```python
from build123d import *

# Parameters (mm, degrees)
F0_W     = 152.095206
F0_H     = 16.764
F1_DEPTH = 254
F2_R     = 9.455493
F2_R_2   = 9.174566
F2_R_3   = 11.28492
F2_R_4   = 9.817554
F3_DEPTH = 203.2


with BuildPart() as f1:
    # F0 (on Front) → F1 (new body)
    with BuildSketch(Plane.XZ):
        with Locations((0.609603, -1.6764)):
            Rectangle(F0_W, F0_H)
    extrude(amount=F1_DEPTH)

    # F2 (on face) → F3 (join)
    with BuildSketch(Plane(origin=(0, 0, -10.0584), x_dir=(1, 0, 0), z_dir=(0, 0, -1))):
        with Locations((-60.858399, 241.452411)):
            Circle(F2_R)
        with Locations((-60.858399, 13.614404)):
            Circle(F2_R_2)
        with Locations((57.353202, 12.954001)):
            Circle(F2_R_3)
        with Locations((56.032401, 243.43361)):
            Circle(F2_R_4)
    extrude(amount=F3_DEPTH)


solid = f1.part
```
Design review of the part built by this model. Coordinates are the model's own, in mm. A direction names the side the tool comes from. Round coordinates to 2 decimals unless told otherwise and drop trailing zeros. Write each loop counter-clockwise with the first axis right and the second up, starting at its lowest first coordinate (ties: lowest second). Pieces come first, ordered by that corner, then holes. Notation, with made-up numbers: (-2.75, 25.5) -> (53.25, 25.5) arc R15 ccw to (53.25, 39.5) -> close; hole circle Ø10 at (35, 60.5). An arc over 180 degrees is marked (long way). Answer in a Markdown table with one row per item.
Q1. Take a section at A-A, the plane x = -57.5. State the section outline as (y, z) points, then the cut area to 3 significant figures.
The answers:
| item | result |
|---|---|
| outline | (-254, -10.06) -> (-250.29, -10.06) -> (-250.29, -213.26) -> (-232.61, -213.26) -> (-232.61, -10.06) -> (-22.15, -10.06) -> (-22.15, -213.26) -> (-5.08, -213.26) -> (-5.08, -10.06) -> (0, -10.06) -> (0, 6.71) -> (-254, 6.71) -> close |
| area | 11,300 mm² |
Q2. Clearance check with flat-ended pins moving along their axes: pin 1 Ø8 at (x, y) = (27.5, -70.5) entering from -Z; pin 2 Ø12 at (y, z) = (-36, -157.5) entering from +X. State where each tip first meets the part, or that it passes through.
The answers:
| item | result |
|---|---|
| pin 1 | z = -10.06 |
| pin 2 | through |
Q3. Take a section at B-B, the plane z = -65.5. State the section outline as (x, y) points, then the cut area to 3 significant figures.
The answers:
| item | result |
|---|---|
| outline | circle Ø18.91 at (-60.86, -241.45); circle Ø18.35 at (-60.86, -13.61); circle Ø22.57 at (57.35, -12.95); circle Ø19.64 at (56.03, -243.43) |
| area | 1,250 mm² |
Q4. For faces 1 (the face through (-52, -16, -110)), 2 (the face through (0, -254, -2)), list the 3-axis set-ups (+Z, -Z, +X, -X, +Y, -Y) from which the entire face can be reached by the end or side of a thin tool; tool diameter is ignored.
The answers:
| item | result |
|---|---|
| face 1 | -Z |
| face 2 | +Z, -Z, +X, -X, -Y |
Q5. Take a section at D-D, the plane x = 23.5. State the section outline as (y, z) points.
The answers:
| item | result |
|---|---|
| outline | (-254, -10.06) -> (0, -10.06) -> (0, 6.71) -> (-254, 6.71) -> close |
Q6. Take a section at C-C, the plane y = -224. State the section outline as (x, z) points.
The answers:
| item | result |
|---|---|
| outline | (-75.44, -10.06) -> (76.66, -10.06) -> (76.66, 6.71) -> (-75.44, 6.71) -> close |
Q7. To check wall thickness, follow L1, parallel to Z at x = -39, y = -106; L2, parallel to Y at x = 51, z = -143; L3, parallel to Y at x = -59.5, z = -139 (3 decimals). State the ranges of each line that lie inside material, in increasing order. Write a range as [from, to].
The answers:
| item | result |
|---|---|
| L1 | [-10.06, 6.71] |
| L2 | [-251.86, -235], [-22.28, -3.63] |
| L3 | [-250.81, -232.095], [-22.688, -4.541] |
Q8. Draft analysis for pull direction Y (two halves, no side actions). For faces 3 (the face through (0, -125, -10.058)), 4 (the face through (56, -244, -213.258)), 5 (the face through (46.08, -13.45, -110.24)), 6 (the face through (0, 0, -2)), state which applies: +Y half, -Y half, draft (parallel to the pull), parting line (faces both ways), or undercut.
The answers:
| item | result |
|---|---|
| face 3 | undercut |
| face 4 | draft |
| face 5 | undercut |
| face 6 | +Y half |
